Here's how the part is built. I have some questions about the finished solid (model axes, mm). A direction names the side the tool comes from. Round coordinates to 2 decimals unless told otherwise and drop trailing zeros. Order: outer loops, then holes, each group sorted by start corner. A loop starts at its lowest first (then second) coordinate and runs counter-clockwise, first axis right, second up. Notation, with made-up numbers: (42, -16.75) -> (78, -16.75) arc R23 cw to (78, 13.25) -> close; hole circle Ø3 at (20.25, 29). An arc over 180 degrees is marked (long way). Use a Markdown table: item, result. Add a question column.
(1) I'm going to push flat-ended pins straight in: P1, Ø10, axis at x = 1.5, z = 148.5, coming from the -Y side; P2, Ø3, axis at y = 11.45, z = 91.67, coming from the +X side; P3, Ø6, axis at x = 9.5, z = 179.5, coming from the -Y side; P4, Ø2.5, axis at y = 19.78, z = 100, coming from the +X side. Where does each tip first touch, or does it pass through?
(2) If I drill on probe 1 along Y at (x, z) = (0, 100); probe 2 along X at (y, z) = (26, 27); probe 3 along Y at (x, z) = (14.25, 172), over which ranges is the centre line in solid material (lowest first)?
(3) I want a section at C-C, the plane x = 6. Please give me the cut outline in (y, z), then the cut area to 3 significant figures.
(4) I want a section at B-B, the plane y = -8. Please give me the cut outline in (x, z), then the cut area to 3 significant figures.
(5) On a 3-axis mill with a long thin cutter (end or side, diameter ignored), from which of +Z, -Z, +X, -X, +Y, -Y can I reach the whole of each face in a straight line? I mean faces 1 (the face through (26, -40, 99)), 2 (the face through (1.5, 2, 99)). Say none if no direction works.
(6) I want a section at A-A, the plane z = 54.5. Please give me the cut outline in (x, y), then the cut area to 3 significant figures.
Autodesk Inventor part; units mm, degrees
ref_plane "YZ Plane" through (0, 0, 0) normal (1, 0, 0) x (0, 1, 0)
ref_plane "XZ Plane" through (0, 0, 0) normal (0, 1, 0) x (-1, 0, 0)
ref_plane "XY Plane" through (0, 0, 0) normal (0, 0, 1) x (1, 0, 0)
sketch "Sketch3" plane through (0, 0, 0) normal (0, 0, 1) x (1, 0, 0)
  line L0 (-1.5, 30.2485) -> (1.5, 30.2485)
  line L1 (1.5, 30.2485) -> (1.5, -30.2485)
  line L2 (1.5, -30.2485) -> (-1.5, -30.2485)
  line L3 (-1.5, -30.2485) -> (-1.5, 30.2485)
  line L4 (1.5, -28.2515) -> (26, -38.4996)
  line L5 (26, -38.4996) -> (26, -41.7515)
  line L6 (26, -41.7515) -> (-1.5, -30.2485)
  point P0 (0, 0)
  point P1 (0, 30.2485)
  point P2 (1.5, 0)
  dimension "d20" = 3
  dimension "d26" = 24.5
  dimension "d39" = 3
  dimension "d41" = 58.5
  dimension "d43" = 72
extrude "Extrusion3" add sketch "Sketch3" along normal blind 200
sketch "Sketch4" plane through (1.5, -28.2515, 0) normal (1, 0, 0) x (0, 0, -1)
  circle A0 centre (-100, 48.031) radius 1.345
  circle A1 centre (-100, 31.369) radius 1.345
  circle A2 centre (-91.669, 39.7) radius 1.345
  circle A3 centre (-108.331, 39.7) radius 1.345
  line L0 (0, 58.5) -> (0, 0)
  line L1 (0, 58.5) -> (-200, 58.5)
  line L2 (-200, 0) -> (-200, 58.5)
  line L3 (0, 0) -> (-200, 0)
  point P0 (-100, 58.5)
  dimension "d28" = 2.69
  dimension "d30" = 8.331
  dimension "d31" = 8.331
  dimension "d32" = 8.331
  dimension "d33" = 8.331
  dimension "d34" = 16.662
  dimension "d35" = 16.662
  dimension "d36" = 10.469
extrude "Extrusion4" cut sketch "Sketch4" against normal through all contours A0 | A1 | A2 | A3
fillet "Fillet1" radius 2 1 edges at (1.5, -28.2515, 100)
equation "\"d31\" = d30"
equation "\"d32\" = d30"
equation "\"d33\" = d30"
equation "\"d35\" = d34"
properties part number "FlatPlow"
Taken from the geometry:
| question | item | result |
|---|---|---|
| 1 | P1 | stops at y = -33.59 |
| 1 | P2 | stops at x = 1.5 |
| 1 | P3 | stops at y = -36.1 |
| 1 | P4 | passes through |
| 2 | probe 1 | y = -30.88 to 1.77, 4.46 to 18.43, 21.12 to 30.25 |
| 2 | probe 2 | x = -1.5 to 1.5 |
| 2 | probe 3 | y = -36.84 to -33.58 |
| 3 | outline | (-33.39, 0) -> (-30.13, 0) -> (-30.13, 200) -> (-33.39, 200) -> close |
| 3 | area | 650 mm2 |
| 4 | outline | (-1.5, 0) -> (1.5, 0) -> (1.5, 200) -> (-1.5, 200) -> close |
| 4 | area | 600 mm2 |
| 5 | face 1 | +Z, -Z, +X, +Y, -Y |
| 5 | face 2 | +Z, -Z, +X, +Y |
| 6 | outline | (-1.5, -30.25) -> (26, -41.75) -> (26, -38.5) -> (2.73, -28.77) arc R2 cw to (1.5, -26.92) -> (1.5, 30.25) -> (-1.5, 30.25) -> close |
| 6 | area | 263 mm2 |
